Source: CAD feature listing. Evaluate the final solid. Frame: model axes, mm. Coordinates: 2 decimals unless noted, no trailing zeros. Order: outer loops, then holes, each group sorted by start corner. A loop starts at its lowest first (then second) coordinate and runs counter-clockwise, first axis right, second up. Notation, with made-up numbers: (-32, 13) - (-20, 13) arc R16 cw to (-20, 24) - close; hole circle Ø6 at (19, -16). An arc over 180 degrees is marked (long way). One line per question, with ' | ' between items.
from build123d import *

# Parameters (mm, degrees)
BOSS_EXTRUDE1_DEPTH = 5


with BuildPart() as part:
    # Sketch1 → Boss-Extrude1 (new body)
    with BuildSketch(Plane(origin=(0, 0, 0), x_dir=(1, 0, 0), z_dir=(0, 1, 0))):
        with BuildLine():
            Line((-1.5, 0), (-2, 0))
            ThreePointArc((-2, 0), (-2.129190076, -0.335410197), (-2.45, -0.497493719))
            ThreePointArc((-2.45, -0.497493719), (-2.309698831, -0.956708581), (-2.084192796, -1.380630432))
            ThreePointArc((-2.084192796, -1.380630432), (-1.414213562, -1.414213562), (-1.380630432, -2.084192796))
            ThreePointArc((-1.380630432, -2.084192796), (-0.956708581, -2.309698831), (-0.497493719, -2.45))
            ThreePointArc((-0.497493719, -2.45), (0, -2), (0.497493719, -2.45))
            ThreePointArc((0.497493719, -2.45), (0.956708581, -2.309698831), (1.380630432, -2.084192796))
            ThreePointArc((1.380630432, -2.084192796), (1.414213562, -1.414213562), (2.084192796, -1.380630432))
            ThreePointArc((2.084192796, -1.380630432), (2.309698831, -0.956708581), (2.45, -0.497493719))
            ThreePointArc((2.45, -0.497493719), (2.129190076, -0.335410197), (2, 0))
            Line((2, 0), (1.5, 0))
            ThreePointArc((1.5, 0), (0, -1.5), (-1.5, 0))
        make_face()
        with BuildLine():
            ThreePointArc((-2.45, 0.497493719), (-2.129190076, 0.335410197), (-2, 0))
            Line((-2, 0), (-1.5, 0))
            ThreePointArc((-1.5, 0), (0, 1.5), (1.5, 0))
            Line((1.5, 0), (2, 0))
            ThreePointArc((2, 0), (2.129190076, 0.335410197), (2.45, 0.497493719))
            ThreePointArc((2.45, 0.497493719), (2.309698831, 0.956708581), (2.084192796, 1.380630432))
            ThreePointArc((2.084192796, 1.380630432), (1.414213562, 1.414213562), (1.380630432, 2.084192796))
            ThreePointArc((1.380630432, 2.084192796), (0.956708581, 2.309698831), (0.497493719, 2.45))
            ThreePointArc((0.497493719, 2.45), (0, 2), (-0.497493719, 2.45))
            ThreePointArc((-0.497493719, 2.45), (-0.956708581, 2.309698831), (-1.380630432, 2.084192796))
            ThreePointArc((-1.380630432, 2.084192796), (-1.414213562, 1.414213562), (-2.084192796, 1.380630432))
            ThreePointArc((-2.084192796, 1.380630432), (-2.309698831, 0.956708581), (-2.45, 0.497493719))
        make_face()
    extrude(amount=BOSS_EXTRUDE1_DEPTH)


solid = part.part
(1) Pull-direction query (X, two-part tool) for faces 1 (the cylindrical face through (0.96, 2.46, -2.31)), 2 (the flat face through (0, 5, -1.7)), 3 (the cylindrical face through (-2.312, 2.465, 0.95)), 4 (the cylindrical face through (0, 2, 2)); classes: pulls with the +X half, pulls with the -X half, needs draft (parallel to the pull), parting line crosses it, or undercut.
Taken from the geometry:
face 1: pulls with the +X half | face 2: needs draft | face 3: pulls with the -X half | face 4: undercut
(2) Pin query (flat end, axial travel): P1, Ø2, axis at y = 4, z = -2, coming from the +X side. Return the tip coordinate at first contact, or that it passes through.
Taken from the geometry:
P1: stops at x = 2.29
(3) Cut plane B-B (x = 0). Return the cut outline in (y, z).
Taken from the geometry:
outline: (0, -2) - (5, -2) - (5, -1.5) - (0, -1.5) - close; (0, 1.5) - (5, 1.5) - (5, 2) - (0, 2) - close
(4) Cut plane C-C (z = 0.2). Return the cut outline in (x, y).
Taken from the geometry:
outline: (-2.04, 0) - (-1.49, 0) - (-1.49, 5) - (-2.04, 5) - close; (1.49, 0) - (2.04, 0) - (2.04, 5) - (1.49, 5) - close
(5) Cut plane A-A (y = 1.3). Return the cut outline in (x, z).
Taken from the geometry:
outline: (-2.45, -0.5) arc R2.5 ccw to (-2.08, -1.38) arc R0.5 cw to (-1.38, -2.08) arc R2.5 ccw to (-0.5, -2.45) arc R0.5 cw to (0.5, -2.45) arc R2.5 ccw to (1.38, -2.08) arc R0.5 cw to (2.08, -1.38) arc R2.5 ccw to (2.45, -0.5) arc R0.5 cw to (2.45, 0.5) arc R2.5 ccw to (2.08, 1.38) arc R0.5 cw to (1.38, 2.08) arc R2.5 ccw to (0.5, 2.45) arc R0.5 cw to (-0.5, 2.45) arc R2.5 ccw to (-1.38, 2.08) arc R0.5 cw to (-2.08, 1.38) arc R2.5 ccw to (-2.45, 0.5) arc R0.5 cw to start; hole circle Ø3 at (0, 0)
(6) Material intervals for L1, parallel to X at y = 4.05, z = 0; L2, parallel to X at y = 1.45, z = -0.8, sorted ascending. Write a range as from..to.
Taken from the geometry:
L1: x = -2..-1.5, 1.5..2 | L2: x = -2.37..-1.27, 1.27..2.37
(7) Cut plane D-D (z = 1.65). Return the cut outline in (x, y), and give its area (3 significant figures).
Taken from the geometry:
outline: (-1.28, 0) - (1.28, 0) - (1.28, 5) - (-1.28, 5) - close | area: 12.8 mm²
